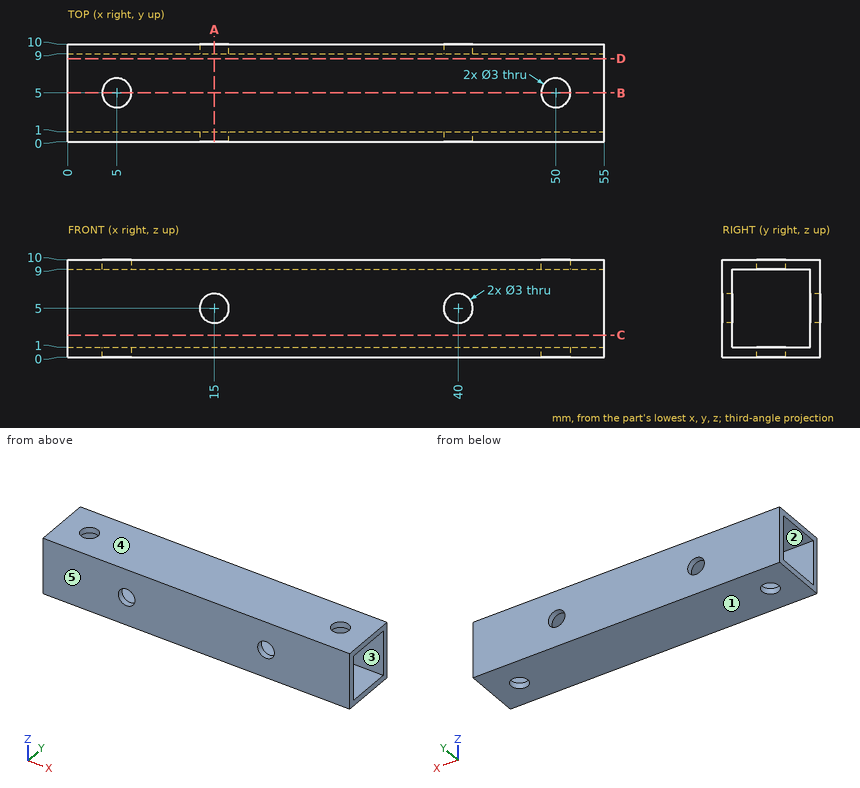
Check sheet for the drawn part. Datum: minimum x, y, z corner. Units: mm. A direction names the side the tool comes from. Coordinates: 2 decimals unless noted, no trailing zeros. Write each loop counter-clockwise with the first axis right and the second up, starting at its lowest first coordinate (ties: lowest second). Pieces come first, ordered by that corner, then holes. Notation, with made-up numbers: M 32,71.5 L 60,71.5 A10 cw 60,79.5 Z; hole C 9.5,81.25 d6. An arc over 180 degrees is marked long. Use a Markdown table: item, result.
Q1. Draft check along Y on the marked faces 3, 4 and 5. Enter one of: +Y half, -Y half, draft (parallel to the pull), parting line (faces both ways), or undercut.
Reply:
| item | result |
|---|---|
| face 3 | undercut |
| face 4 | draft |
| face 5 | -Y half |
Q2. Sectioned sample at A-A, the plane x = 15. Record the boundary of the cut face in (y, z).
Reply:
| item | result |
|---|---|
| outline | M 0,0 L 10,0 L 10,3.5 L 9,3.5 L 9,1 L 1,1 L 1,3.5 L 0,3.5 Z; M 0,6.5 L 1,6.5 L 1,9 L 9,9 L 9,6.5 L 10,6.5 L 10,10 L 0,10 Z |
Q3. Thickness scan on line 1 (Z direction, x = 8.5, y = 1.75); line 2 (Z direction, x = 40, y = 9.65). Record the ranges inside material, lowest first.
Reply:
| item | result |
|---|---|
| line 1 | z = 0 to 1, 9 to 10 |
| line 2 | z = 0 to 3.5, 6.5 to 10 |
Q4. Sectioned sample at C-C, the plane z = 2.25. Record the boundary of the cut face in (x, y).
Reply:
| item | result |
|---|---|
| outline | M 0,0 L 55,0 L 55,1 L 0,1 Z; M 0,9 L 55,9 L 55,10 L 0,10 Z |
Q5. Set-up check for the marked faces 1 and 2: record each of +Z, -Z, +X, -X, +Y, -Y from which the full face is reachable in a straight line by a thin tool's end or side.
Reply:
| item | result |
|---|---|
| face 1 | -Z, +X, -X, +Y, -Y |
| face 2 | +X, -X |
Q6. Sectioned sample at B-B, the plane y = 5. Record the boundary of the cut face in (x, z), plus the area to 3 significant figures.
Reply:
| item | result |
|---|---|
| outline | M 0,0 L 3.5,0 L 3.5,1 L 0,1 Z; M 0,9 L 3.5,9 L 3.5,10 L 0,10 Z; M 6.5,0 L 48.5,0 L 48.5,1 L 6.5,1 Z; M 6.5,9 L 48.5,9 L 48.5,10 L 6.5,10 Z; M 51.5,0 L 55,0 L 55,1 L 51.5,1 Z; M 51.5,9 L 55,9 L 55,10 L 51.5,10 Z |
| area | 98.0 mm² |
